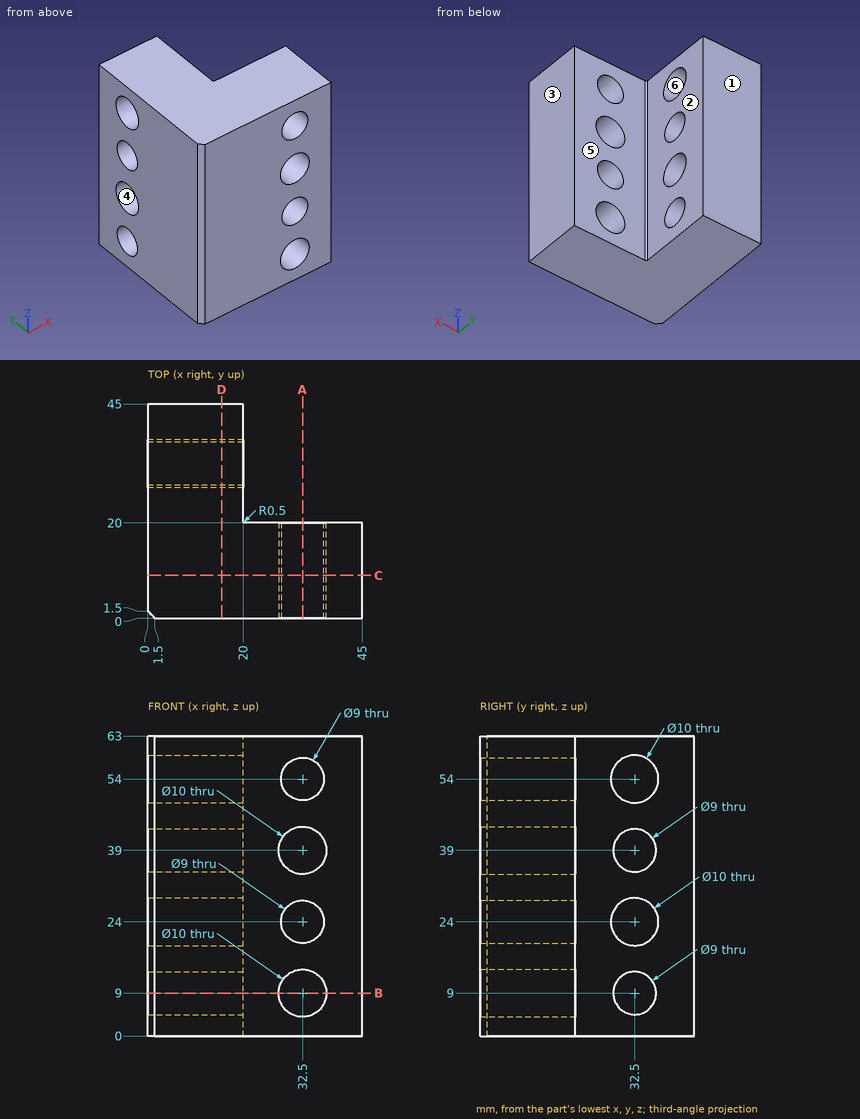
Drawing for the job (mm, zero at the part's lowest x, y, z). A direction names the side the tool comes from. Give positions to 0.01 mm unless a question says otherwise; leave off trailing zeros. Loops run counter-clockwise (first coordinate to the right, second up) from the corner with the lowest first, then second, coordinate; pieces in that order, holes last. Notation, with made-up numbers: M 83,68.5 L 105,68.5 A25 ccw 105,95.5 Z; hole C 38.25,22 d5. An arc over 180 degrees is marked long. One line per question, with ' | ' between items. Start each with the question number.
1. Probe L1, parallel to Z at x = 32.5, y = 10.75; L2, parallel to Z at x = 8, y = 32.5; L3, parallel to X at y = 36, z = 4. List the from-to ranges inside material, lowest first. Write a range as from..to.
2. Saw through at D-D on x = 15.5. Give the cut face in (y, z).
3. Saw through at B-B on z = 9. Give the cut face in (x, y), plus the area to 3 significant figures.
4. Flat gauge pins, fed straight in: pin 1 (8 mm diameter, centred on y = 38.5, z = 11.5, fed in from -X); pin 2 (10.5 mm diameter, centred on x = 32.5, z = 24, fed in from +Y); pin 3 (3 mm diameter, centred on y = 30.5, z = 18, fed in from +X). Where does each tip first touch, or does it go through?
5. Two-plate mould, pull along Y, no slides. Class the marked faces 3, 4, 5 and 6: pulls with the +Y half, pulls with the -Y half, needs draft (parallel to the pull), parting line crosses it, or undercut.
6. Saw through at A-A on x = 32.5. Give the cut face in (y, z), plus the area to 3 significant figures.
7. Saw through at C-C on y = 9. Give the cut face in (x, z).
8. 3-axis set-ups, long thin cutter, end or side, ignore diameter. For the marked faces 1 and 2: which of +Z, -Z, +X, -X, +Y, -Y reach the whole face in a straight line?
Result sheet:
1) L1: z = 0..4, 14..19.5, 28.5..34, 44..49.5, 58.5..63 | L2: z = 0..4.5, 13.5..19, 29..34.5, 43.5..49, 59..63 | L3: x = 0..20
2) outline: M 0,0 L 45,0 L 45,63 L 0,63 Z; hole C 32.5,24 d10; hole C 32.5,54 d10; hole C 32.5,9 d9; hole C 32.5,39 d9
3) outline: M 0,1.5 L 1.5,0 L 27.5,0 L 27.5,20 L 20.5,20 A0.5 cw 20,20.5 L 20,28 L 0,28 Z; M 0,37 L 20,37 L 20,45 L 0,45 Z; M 37.5,0 L 45,0 L 45,20 L 37.5,20 Z | area: 1,020 mm^2
4) pin 1: stops at x = 0 | pin 2: stops at y = 20 | pin 3: stops at x = 20
5) face 3: needs draft | face 4: undercut | face 5: pulls with the +Y half | face 6: undercut
6) outline: M 0,0 L 20,0 L 20,4 L 0,4 Z; M 0,14 L 20,14 L 20,19.5 L 0,19.5 Z; M 0,28.5 L 20,28.5 L 20,34 L 0,34 Z; M 0,44 L 20,44 L 20,49.5 L 0,49.5 Z; M 0,58.5 L 20,58.5 L 20,63 L 0,63 Z | area: 500 mm^2
7) outline: M 0,0 L 45,0 L 45,63 L 0,63 Z; hole C 32.5,9 d10; hole C 32.5,39 d10; hole C 32.5,24 d9; hole C 32.5,54 d9
8) face 1: +Z, -Z, +X, -X, +Y | face 2: +Z, -Z, +X, +Y
